from build123d import *

# Parameters (mm, degrees)
F0_R      = 25.4414928825
F1_DEPTH  = 5
F2_R      = 23.75
F3_DEPTH  = 2
F4_W      = 4.6242554672
F4_H      = 13.1795220077
F5_DEPTH  = 5
F6_R      = 1
F8_D      = 3
F9_W      = 33.4208746554
F9_H      = 3.9936437383
F10_DEPTH = 5
F11_R     = 1.5
F12_R     = 1


with BuildPart() as f1:
    # F0 (on Front) → F1 (new body)
    with BuildSketch(Plane.XZ):
        Circle(F0_R)
    extrude(amount=F1_DEPTH)

    # F2 (on face) → F3 (cut)
    with BuildSketch(Plane.XZ.offset(5)):
        Circle(F2_R)
        with BuildLine():
            add(Edge.make_bspline(
                [(-7.2510674036, -5.9716344181), (-8.0767025075, -6.4364150185), (-9.2574184429, -6.4364150185)],
                knots=[0, 0, 0, 1, 1, 1], degree=2))
            add(Edge.make_bspline(
                [(-9.2574184429, -6.4364150185), (-10.729704817, -6.4364150185), (-11.4687348401, -5.6598561271)],
                knots=[0, 0, 0, 1, 1, 1], degree=2))
            add(Edge.make_bspline(
                [(-11.4687348401, -5.6598561271), (-12.2077648632, -4.8832972356), (-12.2077648632, -3.5293711386)],
                knots=[0, 0, 0, 1, 1, 1], degree=2))
            add(Edge.make_bspline(
                [(-12.2077648632, -3.5293711386), (-12.2077648632, -2.0137822241), (-11.2103630156, -1.2025813003)],
                knots=[0, 0, 0, 1, 1, 1], degree=2))
            add(Edge.make_bspline(
                [(-11.2103630156, -1.2025813003), (-10.212961168, -0.3913803765), (-7.9958710988, -0.336530492)],
                knots=[0, 0, 0, 1, 1, 1], degree=2))
            Line((-7.9958710988, -0.336530492), (-5.8018757177, -0.2990016236))
            Line((-5.8018757177, -0.2990016236), (-5.8018757177, 0.2321762055))
            add(Edge.make_bspline(
                [(-5.8018757177, 0.2321762055), (-5.8018757177, 1.4215526489), (-6.3070720225, 1.9368528798)],
                knots=[0, 0, 0, 1, 1, 1], degree=2))
            add(Edge.make_bspline(
                [(-6.3070720225, 1.9368528798), (-6.8122683274, 2.4521531108), (-7.8948318378, 2.4521531108)],
                knots=[0, 0, 0, 1, 1, 1], degree=2))
            add(Edge.make_bspline(
                [(-7.8948318378, 2.4521531108), (-8.9860558563, 2.4521531108), (-9.482591653, 2.0811946812)],
                knots=[0, 0, 0, 1, 1, 1], degree=2))
            add(Edge.make_bspline(
                [(-9.482591653, 2.0811946812), (-9.9791274498, 1.7102362517), (-10.0801667108, 0.8990353279)],
                knots=[0, 0, 0, 1, 1, 1], degree=2))
            Line((-10.0801667108, 0.8990353279), (-11.774739459, 1.0520376373))
            add(Edge.make_bspline(
                [(-11.774739459, 1.0520376373), (-11.359035071, 3.6877189307), (-7.8601898055, 3.6877189307)],
                knots=[0, 0, 0, 1, 1, 1], degree=2))
            add(Edge.make_bspline(
                [(-7.8601898055, 3.6877189307), (-6.0183884198, 3.6877189307), (-5.0902706369, 2.8433193925)],
                knots=[0, 0, 0, 1, 1, 1], degree=2))
            add(Edge.make_bspline(
                [(-5.0902706369, 2.8433193925), (-4.162152854, 1.9989198544), (-4.162152854, 0.4024995311)],
                knots=[0, 0, 0, 1, 1, 1], degree=2))
            Line((-4.162152854, 0.4024995311), (-4.162152854, -3.8007337252))
            add(Edge.make_bspline(
                [(-4.162152854, -3.8007337252), (-4.162152854, -4.5224427322), (-3.9716216761, -4.8876274897)],
                knots=[0, 0, 0, 1, 1, 1], degree=2))
            add(Edge.make_bspline(
                [(-3.9716216761, -4.8876274897), (-3.7810904983, -5.2528122472), (-3.2499126692, -5.2528122472)],
                knots=[0, 0, 0, 1, 1, 1], degree=2))
            add(Edge.make_bspline(
                [(-3.2499126692, -5.2528122472), (-3.016078951, -5.2528122472), (-2.7187348401, -5.1893018546)],
                knots=[0, 0, 0, 1, 1, 1], degree=2))
            Line((-2.7187348401, -5.1893018546), (-2.7187348401, -6.1996944643))
            add(Edge.make_bspline(
                [(-2.7187348401, -6.1996944643), (-3.330744078, -6.3440362657), (-3.9716216761, -6.3440362657)],
                knots=[0, 0, 0, 1, 1, 1], degree=2))
            add(Edge.make_bspline(
                [(-3.9716216761, -6.3440362657), (-4.8723145168, -6.3440362657), (-5.2836886507, -5.8705951571)],
                knots=[0, 0, 0, 1, 1, 1], degree=2))
            add(Edge.make_bspline(
                [(-5.2836886507, -5.8705951571), (-5.6950627847, -5.3971540486), (-5.7499126692, -4.3867614389)],
                knots=[0, 0, 0, 1, 1, 1], degree=2))
            Line((-5.7499126692, -4.3867614389), (-5.8018757177, -4.3867614389))
            add(Edge.make_bspline(
                [(-5.8018757177, -4.3867614389), (-6.4254322997, -5.5068538176), (-7.2510674036, -5.9716344181)],
                knots=[0, 0, 0, 1, 1, 1], degree=2))
        make_face(mode=Mode.SUBTRACT)
        with BuildLine():
            add(Edge.make_bspline(
                [(-15.3659634775, -5.3755027784), (-16.3676955791, -6.4364150185), (-18.1084577038, -6.4364150185)],
                knots=[0, 0, 0, 1, 1, 1], degree=2))
            add(Edge.make_bspline(
                [(-18.1084577038, -6.4364150185), (-21.3388272188, -6.4364150185), (-21.9421759486, -3.0963457345)],
                knots=[0, 0, 0, 1, 1, 1], degree=2))
            Line((-21.9421759486, -3.0963457345), (-20.2562637085, -2.8163226398))
            add(Edge.make_bspline(
                [(-20.2562637085, -2.8163226398), (-20.0917140549, -3.8642441178), (-19.5244507754, -4.4502718315)],
                knots=[0, 0, 0, 1, 1, 1], degree=2))
            add(Edge.make_bspline(
                [(-19.5244507754, -4.4502718315), (-18.957187496, -5.0362995451), (-18.0997971958, -5.0362995451)],
                knots=[0, 0, 0, 1, 1, 1], degree=2))
            add(Edge.make_bspline(
                [(-18.0997971958, -5.0362995451), (-17.1615754867, -5.0362995451), (-16.6202937316, -4.3910916929)],
                knots=[0, 0, 0, 1, 1, 1], degree=2))
            add(Edge.make_bspline(
                [(-16.6202937316, -4.3910916929), (-16.0790119764, -3.7458838407), (-16.0790119764, -2.5016575128)],
                knots=[0, 0, 0, 1, 1, 1], degree=2))
            Line((-16.0790119764, -2.5016575128), (-16.0790119764, 5.0503055357))
            Line((-16.0790119764, 5.0503055357), (-18.5241620918, 5.0503055357))
            Line((-18.5241620918, 5.0503055357), (-18.5241620918, 6.4561946812))
            Line((-18.5241620918, 6.4561946812), (-14.3642313759, 6.4561946812))
            Line((-14.3642313759, 6.4561946812), (-14.3642313759, -2.4641286444))
            add(Edge.make_bspline(
                [(-14.3642313759, -2.4641286444), (-14.3642313759, -4.3145905382), (-15.3659634775, -5.3755027784)],
                knots=[0, 0, 0, 1, 1, 1], degree=2))
        make_face(mode=Mode.SUBTRACT)
        with BuildLine():
            add(Edge.make_bspline(
                [(6.7500873308, 4.6519221639), (5.7714499174, 5.2379498775), (4.4261843285, 5.2379498775)],
                knots=[0, 0, 0, 1, 1, 1], degree=2))
            add(Edge.make_bspline(
                [(4.4261843285, 5.2379498775), (2.3159071922, 5.2379498775), (1.142408347, 3.8811369445)],
                knots=[0, 0, 0, 1, 1, 1], degree=2))
            add(Edge.make_bspline(
                [(1.142408347, 3.8811369445), (-0.0310904983, 2.5243240115), (-0.0310904983, 0.1600053048)],
                knots=[0, 0, 0, 1, 1, 1], degree=2))
            add(Edge.make_bspline(
                [(-0.0310904983, 0.1600053048), (-0.0310904983, -2.1754450416), (1.1914845594, -3.5972117853)],
                knots=[0, 0, 0, 1, 1, 1], degree=2))
            add(Edge.make_bspline(
                [(1.1914845594, -3.5972117853), (2.4140596172, -5.0189785289), (4.4983552292, -5.0189785289)],
                knots=[0, 0, 0, 1, 1, 1], degree=2))
            add(Edge.make_bspline(
                [(4.4983552292, -5.0189785289), (7.1686785548, -5.0189785289), (8.5139441437, -2.3746367275)],
                knots=[0, 0, 0, 1, 1, 1], degree=2))
            Line((8.5139441437, -2.3746367275), (9.9198332892, -3.0790247183))
            add(Edge.make_bspline(
                [(9.9198332892, -3.0790247183), (9.1346138897, -4.7216344181), (7.7142905641, -5.5790247183)],
                knots=[0, 0, 0, 1, 1, 1], degree=2))
            add(Edge.make_bspline(
                [(7.7142905641, -5.5790247183), (6.2939672384, -6.4364150185), (4.4175238204, -6.4364150185)],
                knots=[0, 0, 0, 1, 1, 1], degree=2))
            add(Edge.make_bspline(
                [(4.4175238204, -6.4364150185), (2.494891026, -6.4364150185), (1.0918887165, -5.6367614389)],
                knots=[0, 0, 0, 1, 1, 1], degree=2))
            add(Edge.make_bspline(
                [(1.0918887165, -5.6367614389), (-0.311113593, -4.8371078592), (-1.045813362, -3.3532741409)],
                knots=[0, 0, 0, 1, 1, 1], degree=2))
            add(Edge.make_bspline(
                [(-1.045813362, -3.3532741409), (-1.7805131311, -1.8694404227), (-1.7805131311, 0.1600053048)],
                knots=[0, 0, 0, 1, 1, 1], degree=2))
            add(Edge.make_bspline(
                [(-1.7805131311, 0.1600053048), (-1.7805131311, 3.199843642), (-0.1379034313, 4.9232847505)],
                knots=[0, 0, 0, 1, 1, 1], degree=2))
            add(Edge.make_bspline(
                [(-0.1379034313, 4.9232847505), (1.5047062684, 6.6467258591), (4.4088633123, 6.6467258591)],
                knots=[0, 0, 0, 1, 1, 1], degree=2))
            add(Edge.make_bspline(
                [(4.4088633123, 6.6467258591), (6.4383090398, 6.6467258591), (7.8008956449, 5.8528459514)],
                knots=[0, 0, 0, 1, 1, 1], degree=2))
            add(Edge.make_bspline(
                [(7.8008956449, 5.8528459514), (9.16348225, 5.0589660438), (9.8043598481, 3.4971877528)],
                knots=[0, 0, 0, 1, 1, 1], degree=2))
            Line((9.8043598481, 3.4971877528), (8.1704106564, 2.9573494156))
            add(Edge.make_bspline(
                [(8.1704106564, 2.9573494156), (7.7287247442, 4.0658944503), (6.7500873308, 4.6519221639)],
                knots=[0, 0, 0, 1, 1, 1], degree=2))
        make_face(mode=Mode.SUBTRACT)
        Polygon((21.4873852523, 5.0503055357), (17.1196023424, 5.0503055357), (17.1196023424, -6.2545443488), (15.4048217419, -6.2545443488), (15.4048217419, 5.0503055357), (11.039925668, 5.0503055357), (11.039925668, 6.4561946812), (21.4873852523, 6.4561946812), align=None, mode=Mode.SUBTRACT)
    extrude(amount=-F3_DEPTH, mode=Mode.SUBTRACT)

    # F4 (on face) → F5 (join)
    with BuildSketch(Plane(origin=(0, 0, 0), x_dir=(-1, 0, 0), z_dir=(0, 1, 0))):
        with Locations((8.8527675252, 6.5897610039)):
            Rectangle(F4_W, F4_H)
    extrude(amount=F5_DEPTH)

    # F6
    f6_edges = [f1.edges().sort_by_distance(p)[0] for p in [
        (-8.852768, 5, 13.179522),
        (-6.54064, 5, 6.589761),
        (-8.852768, 5, 0),
        (-11.164895, 5, 6.589761),
    ]]
    fillet(f6_edges, radius=F6_R)

    # F8 (through all)
    with Locations(Plane(origin=(0, 0, 0), x_dir=(1, 0, 0), z_dir=(0, 0, -1))):
        with Locations((-8.9718680829, -1.9239948597)):
            Hole(F8_D / 2)

    # F9 (on face) → F10 (join)
    with BuildSketch(Plane(origin=(0, 0, 0), x_dir=(-1, 0, 0), z_dir=(0, 1, 0))):
        with Locations((0, -17.1873081453)):
            Rectangle(F9_W, F9_H)
    extrude(amount=F10_DEPTH)

    # F11
    f11_edges = [f1.edges().sort_by_distance(p)[0] for p in [
        (0, 5, -15.190486),
        (0, 5, -19.18413),
    ]]
    fillet(f11_edges, radius=F11_R)

    # F12
    f12_edges = [f1.edges().sort_by_distance(p)[0] for p in [
        (16.710437, 5, -17.187308),
        (-16.710437, 5, -17.187308),
    ]]
    fillet(f12_edges, radius=F12_R)


solid = f1.part
Geometry check sheet. Reference: the model listing, model coordinates, mm. A direction names the side the tool comes from. Round coordinates to 2 decimals unless told otherwise and drop trailing zeros. Answer in a Markdown table with one row per item.
(1) Sectioned sample at A-A, the plane y = -3.75. State how many separate pieces and enclosed holes the cut face has, and give its area (3 significant figures).
Responses:
| item | result |
|---|---|
| separate pieces | 5 |
| enclosed holes | 1 |
| area | 434 mm² |
(2) Tool access check on faces 4 (the face through (-16.71, 2, -17)), 5 (the face through (9, -4.01, 3.23)), 6 (the face through (0, 2, -19.184)), 7 (the face through (16.71, 2, -17)). Record the directions out of +Z, -Z, +X, -X, +Y, -Y that give a thin tool (end or side, any length) a straight path to the whole face; none if there is none.
Responses:
| item | result |
|---|---|
| face 4 | +Z, -Z, -X, +Y |
| face 5 | -Y |
| face 6 | -Z, +X, -X, +Y |
| face 7 | +Z, -Z, +X, +Y |
(3) Go/stop test with flat-tipped pins: P1, Ø4, axis at x = -0.5, y = 2.5, coming from the +Z side; P2, Ø2, axis at x = -18.5, y = -3, coming from the +Z side; P3, Ø2, axis at y = -4, z = -3.5, coming from the +X side. Record where each tip stops, or that it passes through.
Responses:
| item | result |
|---|---|
| P1 | stops at z = -15.19 |
| P2 | stops at z = 18.47 |
| P3 | stops at x = 25.32 |
(4) Scan lines: probe 1 along Z at (x, y) = (14, -3.75); probe 2 along Z at (x, y) = (-7.5, 3.5); probe 3 along X at (y, z) = (3.75, 11). Record each from-to range of solid material in increasing order. Write a range as from..to.
Responses:
| item | result |
|---|---|
| probe 1 | z = -21.24..-19.18, 5.05..6.46, 19.18..21.24 |
| probe 2 | z = -19.18..-15.19, 0..13.18 |
| probe 3 | x = -11.16..-6.54 |
(5) Draft check along Z on faces 1 (the face through (-15.9, -5, -1.4)), 2 (the face through (-7, 2, 13.18)), 3 (the face through (13, -4, 5.05)). Enter one of: released by +Z, released by -Z, zero draft, split by the parting line, or undercut.
Responses:
| item | result |
|---|---|
| face 1 | zero draft |
| face 2 | released by +Z |
| face 3 | undercut |
